from build123d import *

# Parameters (mm, degrees)
SKETCH_1_R      = 17.7
SKETCH_1_R_2    = 1.65
EXTRUDE_1_DEPTH = 3


with BuildPart() as part:
    # Sketch 1 → Extrude 1 (new body)
    with BuildSketch(Plane.XY):
        with BuildLine():
            ThreePointArc((3, 28), (0, 31), (-3, 28))
            Line((-3, 28), (-3, 20.784609691))
            ThreePointArc((-3, 20.784609691), (-14.935576159, 14.762403761), (-20.818181818, 2.757409252))
            ThreePointArc((-20.818181818, 2.757409252), (-25, 0), (-20.818181818, -2.757409252))
            ThreePointArc((-20.818181818, -2.757409252), (-14.935576159, -14.762403761), (-3, -20.784609691))
            Line((-3, -20.784609691), (-3, -28))
            ThreePointArc((-3, -28), (0, -31), (3, -28))
            Line((3, -28), (3, -20.784609691))
            ThreePointArc((3, -20.784609691), (14.935576159, -14.762403761), (20.818181818, -2.757409252))
            ThreePointArc((20.818181818, -2.757409252), (25, 0), (20.818181818, 2.757409252))
            ThreePointArc((20.818181818, 2.757409252), (14.935576159, 14.762403761), (3, 20.784609691))
            Line((3, 20.784609691), (3, 28))
        make_face()
        Circle(SKETCH_1_R, mode=Mode.SUBTRACT)
        with Locations((0, 28)):
            Circle(SKETCH_1_R_2, mode=Mode.SUBTRACT)
        with Locations((-22, 0)):
            Circle(SKETCH_1_R_2, mode=Mode.SUBTRACT)
        with Locations((22, 0)):
            Circle(SKETCH_1_R_2, mode=Mode.SUBTRACT)
        with Locations((0, -28)):
            Circle(SKETCH_1_R_2, mode=Mode.SUBTRACT)
    extrude(amount=EXTRUDE_1_DEPTH)


solid = part.part
Read the model definition and answer for the solid it produces. Units are mm, in the model's axes. A direction names the side the tool comes from. Give positions to 0.01 mm unless a question says otherwise; leave off trailing zeros. Write each loop counter-clockwise with the first axis right and the second up, starting at its lowest first coordinate (ties: lowest second). Pieces come first, ordered by that corner, then holes. Notation, with made-up numbers: (2.5, -36) - (24.5, -36) arc R27 ccw to (24.5, -11) - close; hole circle Ø1 at (-30.75, 44.5). An arc over 180 degrees is marked (long way). Use CSV: the item, a comma, the result in double quotes. Start each with the question number.
Item 1: For faces 1 (the flat face through (-3, -24, 1)), 2 (the cylindrical face through (-0.215, 29.636, 1.479)), 3 (the flat face through (3, -24, 1)), determine the directions among +Z, -Z, +X, -X, +Y, -Y from which every point of the face is accessible in a straight line to the end or side of a thin tool.
Item 2: Consider line 1 (Y direction, x = 22, z = 1); line 2 (Y direction, x = 0.5, z = 2.75); line 3 (X direction, y = 11, z = 2.15). Determine where each line is inside the solid, lowest interval first.
Item 3: The part is cut by section B-B, the plane z = 0.65. Give the vertices of the cut face in (x, y).
Item 4: The part is cut by section D-D, the plane y = -25. Give the vertices of the cut face in (x, z).
Item 5: Flat-ended cylindrical pins translate along their axes: P1, Ø1.5, axis at y = -26, z = 1.5, coming from the +X side; P2, Ø1.5, axis at y = 22.5, z = 1, coming from the -X side; P3, Ø3, axis at x = 0, y = -28, coming from the +Z side (1 decimal). Find the tip coordinate at first contact, or state that the pin passes through.
Item 6: The part is cut by section A-A, the plane x = 0. Give the vertices of the cut face in (y, z), and give its area (3 significant figures).
Item 7: The mould has two halves that part along X. Classify faces 4 (the cylindrical face through (-23.65, 0.07, 1.48)), 5 (the cylindrical face through (25, 0, 1)), 6 (the flat face through (3, 24, 1)), 7 (the flat face through (-3, 24, 1)): pulls with the +X half, pulls with the -X half, needs draft (parallel to the pull), parting line crosses it, or undercut.
Item 8: The part is cut by section C-C, the plane x = -22. Give the vertices of the cut face in (y, z).
Taken from the geometry:
1,face 1,"+Z, -Z, -X, -Y"
1,face 2,"+Z, -Z"
1,face 3,"+Z, -Z, +X, -Y"
2,line 1,"-3 to -1.65, 1.65 to 3"
2,line 2,"-30.96 to -29.57, -26.43 to -17.69, 17.69 to 26.43, 29.57 to 30.96"
2,line 3,"-17.89 to -13.87, 13.87 to 17.89"
3,outline,"(-20.82, -2.76) arc R21 ccw to (-3, -20.78) - (-3, -28) arc R3 ccw to (3, -28) - (3, -20.78) arc R21 ccw to (20.82, -2.76) arc R3 ccw (long way) to (20.82, 2.76) arc R21 ccw to (3, 20.78) - (3, 28) arc R3 ccw to (-3, 28) - (-3, 20.78) arc R21 ccw to (-20.82, 2.76) arc R3 ccw (long way) to start; hole circle Ø3.3 at (-22, 0); hole circle Ø35.4 at (0, 0); hole circle Ø3.3 at (0, -28); hole circle Ø3.3 at (0, 28); hole circle Ø3.3 at (22, 0)"
4,outline,"(-3, 0) - (3, 0) - (3, 3) - (-3, 3) - close"
5,P1,"x = 3"
5,P2,"x = -3"
5,P3,"through"
6,outline,"(-31, 0) - (-29.65, 0) - (-29.65, 3) - (-31, 3) - close; (-26.35, 0) - (-17.7, 0) - (-17.7, 3) - (-26.35, 3) - close; (17.7, 0) - (26.35, 0) - (26.35, 3) - (17.7, 3) - close; (29.65, 0) - (31, 0) - (31, 3) - (29.65, 3) - close"
6,area,"60.0 mm2"
7,face 4,"undercut"
7,face 5,"undercut"
7,face 6,"pulls with the +X half"
7,face 7,"pulls with the -X half"
8,outline,"(-3, 0) - (-1.65, 0) - (-1.65, 3) - (-3, 3) - close; (1.65, 0) - (3, 0) - (3, 3) - (1.65, 3) - close"
